from build123d import *

# Parameters (mm, degrees)
SKETCH002_R      = 4
EXTRUDE002_DEPTH = 30
SKETCH001_R      = 4
EXTRUDE001_DEPTH = 30
SKETCH_R         = 11
EXTRUDE_DEPTH    = 10


with BuildPart() as extrude002:
    # Sketch002 (on Face1 of Cut) → Extrude002 (new body)
    with BuildSketch(Plane.XY.offset(30)):
        with Locations((2, 0)):
            Circle(SKETCH002_R)
        with Locations((-32, 0)):
            Circle(SKETCH002_R)
    extrude(amount=-EXTRUDE002_DEPTH)


with BuildPart() as extrude001:
    # Sketch001 (on Face6 of Extrude) → Extrude001 (new body)
    with BuildSketch(Plane(origin=(0, 0, -30), x_dir=(1, 0, 0), z_dir=(0, 0, -1))):
        with Locations((-15, 0)):
            Circle(SKETCH001_R)
    extrude(amount=-EXTRUDE001_DEPTH)


with BuildPart() as body:
    # Sketch → Extrude (new body, symmetric)
    with BuildSketch(Plane(origin=(-15, 0, -30), x_dir=(1, 0, 0), z_dir=(0, -1, 0))):
        with BuildLine():
            Line((-22.179407, 60), (22.179407, 60))
            ThreePointArc((25, 56.773532), (24.322176, 59.027097), (22.179407, 60))
            Line((25, 56.773532), (20, 19.694224))
            Line((20, 19.694224), (15, 14.141195))
            Line((15, 14.141195), (15, 0))
            Line((15, 0), (-15, 0))
            Line((-15, 0), (-15, 14.141195))
            Line((-15, 14.141195), (-20, 19.694224))
            Line((-20, 19.694224), (-25, 56.773532))
            ThreePointArc((-22.179407, 60), (-24.322176, 59.027097), (-25, 56.773532))
        make_face()
        with Locations((0, 36.968787)):
            Circle(SKETCH_R, mode=Mode.SUBTRACT)
    extrude(amount=EXTRUDE_DEPTH, both=True)

    # Cut: cut Extrude001
    add(extrude001.part, mode=Mode.SUBTRACT)

    # Cut001: cut Extrude002
    add(extrude002.part, mode=Mode.SUBTRACT)


solid = body.part
Check sheet for the modelled part. Datum: model origin and axes. Units: mm. A direction names the side the tool comes from. Round coordinates to 2 decimals unless told otherwise and drop trailing zeros. Loops run counter-clockwise (first coordinate to the right, second up) from the corner with the lowest first, then second, coordinate; pieces in that order, holes last.
1. Sectioned sample at D-D on x = -10. Record the boundary of the cut face in (y, z), and give its area (3 significant figures).
2. Gauge pin test, flat ends, axial feed: pin 1 Ø10 at (y, z) = (5.5, -5) entering from -X; pin 2 Ø4 at (x, y) = (-32, -1) entering from +Z; pin 3 Ø11.5 at (y, z) = (0.5, -23.5) entering from -X. Record the tip position at first contact, or that the pin passes through.
3. Sectioned sample at A-A on z = -19. Record the boundary of the cut face in (x, y).
4. Scan lines: probe 1 along Y at (x, z) = (-32, 7.5); probe 2 along Z at (x, y) = (-15, 4.5); probe 3 along X at (y, z) = (3.5, 6.5). Record each from-to range of solid material in increasing order.
5. Mould release check, pull along X, two halves, no side actions. Record for faces 1 (the flat face through (0, 0, -23)), 2 (the cylindrical face through (-19, 0, -17)), 3 (the flat face through (-15, 0, 30)): released by +X, released by -X, zero draft, split by the parting line, or undercut.
6. Sectioned sample at C-C on x = -17.5. Record the boundary of the cut face in (y, z).
7. Set-up check for faces 4 (the flat face through (-30, 0, -23)), 5 (the flat face through (2, 0, 0)), 6 (the flat face through (-15, 10, -6)): record each of +Z, -Z, +X, -X, +Y, -Y from which the full face is reachable in a straight line by a thin tool's end or side.
8. Sectioned sample at B-B on y = 0. Record the boundary of the cut face in (x, z), and give its area (3 significant figures).
Recorded:
1. outline: (-10, -30) - (10, -30) - (10, -2.83) - (-10, -2.83) - close; (-10, 16.77) - (10, 16.77) - (10, 30) - (-10, 30) - close
1. area: 808 mm2
2. pin 1: stops at x = -36.39
2. pin 2: stops at z = 0
2. pin 3: stops at x = -30
3. outline: (-30, -10) - (0, -10) - (0, 10) - (-30, 10) - close; hole circle Ø8 at (-15, 0)
4. probe 1: y = -10 to -4, 4 to 10
4. probe 2: z = -30 to -4.03, 17.97 to 30
4. probe 3: x = -37.27 to -33.94, -30.06 to -25.99, -4.01 to 0.06, 3.94 to 7.27
5. face 1: released by +X
5. face 2: undercut
5. face 3: zero draft
6. outline: (-10, -30) - (-3.12, -30) - (-3.12, -3.74) - (-10, -3.74) - close; (-10, 17.68) - (10, 17.68) - (10, 30) - (-10, 30) - close; (3.12, -30) - (10, -30) - (10, -3.74) - (3.12, -3.74) - close
7. face 4: -Z, -X, +Y, -Y
7. face 5: +Z
7. face 6: +Z, -Z, +X, -X, +Y
8. outline: (-40, 26.77) - (-35, -10.31) - (-30, -15.86) - (-30, -30) - (-19, -30) - (-19, -3.28) arc R11 cw (long way) to (-11, -3.28) - (-11, -30) - (0, -30) - (0, -15.86) - (5, -10.31) - (10, 26.77) arc R2.85 ccw to (7.18, 30) - (6, 30) - (6, 0) - (-2, 0) - (-2, 30) - (-28, 30) - (-28, 0) - (-36, 0) - (-36, 30) - (-37.18, 30) arc R2.85 ccw to start
8. area: 1,380 mm2
